Geometry: final body of the model. Coordinates: model frame, mm. Give positions to 0.01 mm unless a question says otherwise; leave off trailing zeros. Write each loop counter-clockwise with the first axis right and the second up, starting at its lowest first coordinate (ties: lowest second). Pieces come first, ordered by that corner, then holes. Notation, with made-up numbers: (-21, -11) -> (-7, -11) arc R29 cw to (-7, 16) -> close; hole circle Ø3 at (-23.75, 11). An arc over 180 degrees is marked (long way). Answer as a JSON object with one key per item and string values. Group by question number.
(1) Section query B-B on x = 60.3. Output: boundary loops of the cut face in (y, z).
(2) Section query D-D on z = -3.2. Output: boundary loops of the cut face in (x, y), plus the area to 4 significant figures.
(3) Section query C-C on z = -10. Output: boundary loops of the cut face in (x, y) (3 decimals).
(4) Material intervals for probe 1 along X at (y, z) = (1.1, -50); probe 2 along Z at (x, y) = (30, 0.75); probe 3 along X at (y, z) = (0.75, -17) (3 decimals), sorted ascending.
(5) Contact query for a flat-ended pin moving along its axis: pin 1 Ø4.5 at (x, z) = (3, -60) entering from +Y. Output: stop coordinate, or through.
(6) Section query A-A on z = -50.5. Output: boundary loops of the cut face in (x, y).
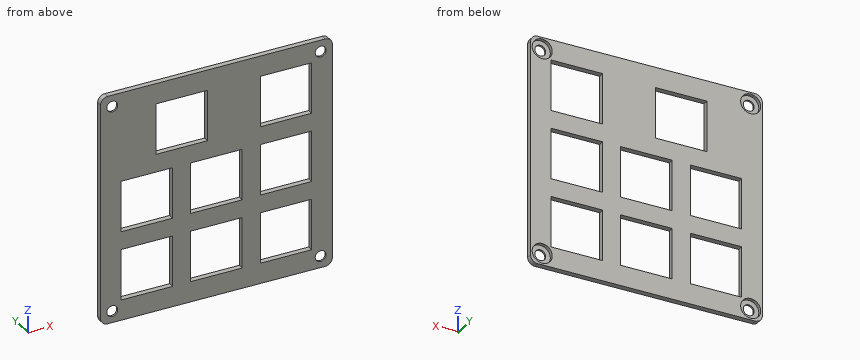
from build123d import *

# Parameters (mm, degrees)
SKETCH1_W           = 63.5
SKETCH1_H           = 63.5
BOSS_EXTRUDE1_DEPTH = 1.5
SKETCH2_R           = 1.5
SKETCH2_W           = 14.1
SKETCH2_H           = 14.1
CUT_EXTRUDE1_DEPTH  = 90.815087819
SKETCH4_R           = 2.75
CUT_EXTRUDE2_DEPTH  = 1
FILLET1_R           = 2


with BuildPart() as part:
    # Sketch1 → Boss-Extrude1 (new body)
    with BuildSketch(Plane(origin=(0, 0, 0), x_dir=(1, 0, 0), z_dir=(0, 1, 0))):
        with Locations((31.75, 31.75)):
            Rectangle(SKETCH1_W, SKETCH1_H)
    extrude(amount=BOSS_EXTRUDE1_DEPTH)

    # Sketch2 → Cut-Extrude1 (cut, through all)
    with BuildSketch(Plane(origin=(0, 1.5, 0), x_dir=(1, 0, 0), z_dir=(0, 1, 0))):
        with Locations(Location((3.2, 60.3, 0), (0, 0, 270))):
            Circle(SKETCH2_R)
        with Locations(Location((60.3, 60.3, 0), (0, 0, 270))):
            Circle(SKETCH2_R)
        with Locations(Location((60.3, 3.2, 0), (0, 0, 270))):
            Circle(SKETCH2_R)
        with Locations(Location((3.2, 3.2, 0), (0, 0, 270))):
            Circle(SKETCH2_R)
        with Locations((12.7, 50.8)):
            Rectangle(SKETCH2_W, SKETCH2_H)
        with Locations((31.75, 50.8)):
            Rectangle(SKETCH2_W, SKETCH2_H)
        with Locations((50.8, 50.8)):
            Rectangle(SKETCH2_W, SKETCH2_H)
        with Locations((12.7, 31.75)):
            Rectangle(SKETCH2_W, SKETCH2_H)
        with Locations((31.75, 31.75)):
            Rectangle(SKETCH2_W, SKETCH2_H)
        with Locations((50.8, 31.75)):
            Rectangle(SKETCH2_W, SKETCH2_H)
        with Locations((22.225, 12.7)):
            Rectangle(SKETCH2_W, SKETCH2_H)
        with Locations((50.8, 12.7)):
            Rectangle(SKETCH2_W, SKETCH2_H)
    extrude(amount=-CUT_EXTRUDE1_DEPTH, mode=Mode.SUBTRACT)

    # Sketch4 → Cut-Extrude2 (cut)
    with BuildSketch(Plane(origin=(0, 1.5, 0), x_dir=(1, 0, 0), z_dir=(0, 1, 0))):
        with Locations(Location((3.2, 60.3, 0), (0, 0, 270))):
            Circle(SKETCH4_R)
        with Locations(Location((60.3, 60.3, 0), (0, 0, 270))):
            Circle(SKETCH4_R)
        with Locations(Location((60.3, 3.2, 0), (0, 0, 270))):
            Circle(SKETCH4_R)
        with Locations(Location((3.2, 3.2, 0), (0, 0, 270))):
            Circle(SKETCH4_R)
    extrude(amount=-CUT_EXTRUDE2_DEPTH, mode=Mode.SUBTRACT)

    # Fillet1
    fillet1_edges = [part.edges().sort_by_distance(p)[0] for p in [
        (0, 0.75, -63.5),
        (63.5, 0.75, -63.5),
        (63.5, 0.75, 0),
        (0, 0.75, 0),
    ]]
    fillet(fillet1_edges, radius=FILLET1_R)


solid = part.part
Answer list:
{
 "1": {"outline": "(0, -63.5) -> (1.5, -63.5) -> (1.5, -63.05) -> (0.5, -63.05) -> (0.5, -61.8) -> (0, -61.8) -> close; (0, -58.8) -> (0.5, -58.8) -> (0.5, -57.55) -> (1.5, -57.55) -> (1.5, -5.95) -> (0.5, -5.95) -> (0.5, -4.7) -> (0, -4.7) -> close; (0, -1.7) -> (0.5, -1.7) -> (0.5, -0.45) -> (1.5, -0.45) -> (1.5, 0) -> (0, 0) -> close"},
 "2": {"outline": "(0, 0) -> (1.7, 0) -> (1.7, 0.5) -> (0.45, 0.5) -> (0.45, 1.5) -> (0, 1.5) -> close; (4.7, 0) -> (58.8, 0) -> (58.8, 0.5) -> (57.55, 0.5) -> (57.55, 1.5) -> (5.95, 1.5) -> (5.95, 0.5) -> (4.7, 0.5) -> close; (61.8, 0) -> (63.5, 0) -> (63.5, 1.5) -> (63.05, 1.5) -> (63.05, 0.5) -> (61.8, 0.5) -> close", "area": "81.25 mm2"},
 "3": {"outline": "(0, 0) -> (15.175, 0) -> (15.175, 1.5) -> (0, 1.5) -> close; (29.275, 0) -> (43.75, 0) -> (43.75, 1.5) -> (29.275, 1.5) -> close; (57.85, 0) -> (63.5, 0) -> (63.5, 1.5) -> (57.85, 1.5) -> close"},
 "4": {"probe 1": "0 to 5.65, 19.75 to 24.7, 38.8 to 43.75, 57.85 to 63.5", "probe 2": "-63.5 to -57.85, -43.75 to -38.8, -24.7 to 0", "probe 3": "0 to 15.175, 29.275 to 43.75, 57.85 to 63.5"},
 "5": {"pin 1": "y = 0.5"},
 "6": {"outline": "(0, 0) -> (5.65, 0) -> (5.65, 1.5) -> (0, 1.5) -> close; (19.75, 0) -> (24.7, 0) -> (24.7, 1.5) -> (19.75, 1.5) -> close; (38.8, 0) -> (43.75, 0) -> (43.75, 1.5) -> (38.8, 1.5) -> close; (57.85, 0) -> (63.5, 0) -> (63.5, 1.5) -> (57.85, 1.5) -> close"}
}
